```python
from build123d import *

# Parameters (mm, degrees)
BOSS_EXTRUDE1_DEPTH = 25.4
SKETCH2_R           = 1.0287
BOSS_EXTRUDE2_DEPTH = 6.35
SKETCH3_R           = 1.0287
CUT_EXTRUDE1_DEPTH  = 6.35


with BuildPart() as part:
    # Sketch1 → Boss-Extrude1 (new body)
    with BuildSketch(Plane(origin=(0, 0, 0), x_dir=(1, 0, 0), z_dir=(0, 1, 0))):
        with BuildLine():
            Line((-1.135922533, 2.413), (1.135922533, 2.413))
            ThreePointArc((1.135922533, 2.413), (1.3335, 2.309689752), (1.521758033, 2.19023777))
            Line((1.521758033, 2.19023777), (2.657680566, 0.22276223))
            ThreePointArc((2.657680566, 0.22276223), (2.667, 0), (2.657680566, -0.22276223))
            Line((2.657680566, -0.22276223), (1.521758033, -2.19023777))
            ThreePointArc((1.521758033, -2.19023777), (1.3335, -2.309689752), (1.135922533, -2.413))
            Line((1.135922533, -2.413), (-1.135922533, -2.413))
            ThreePointArc((-1.135922533, -2.413), (-1.3335, -2.309689752), (-1.521758033, -2.19023777))
            Line((-1.521758033, -2.19023777), (-2.657680566, -0.22276223))
            ThreePointArc((-2.657680566, -0.22276223), (-2.667, 0), (-2.657680566, 0.22276223))
            Line((-2.657680566, 0.22276223), (-1.521758033, 2.19023777))
            ThreePointArc((-1.521758033, 2.19023777), (-1.3335, 2.309689752), (-1.135922533, 2.413))
        make_face()
    extrude(amount=BOSS_EXTRUDE1_DEPTH)

    # Sketch2 → Boss-Extrude2 (add)
    with BuildSketch(Plane(origin=(0, 25.4, 0), x_dir=(1, 0, 0), z_dir=(0, 1, 0))):
        Circle(SKETCH2_R)
    extrude(amount=BOSS_EXTRUDE2_DEPTH)

    # Sketch3 → Cut-Extrude1 (cut)
    with BuildSketch(Plane.XZ):
        Circle(SKETCH3_R)
    extrude(amount=-CUT_EXTRUDE1_DEPTH, mode=Mode.SUBTRACT)


solid = part.part
```
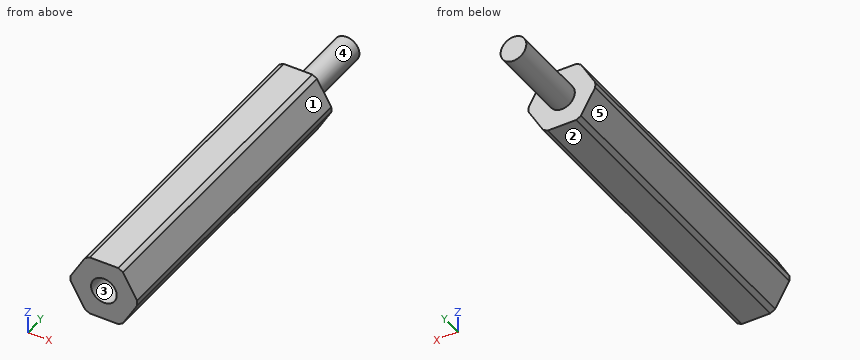
Part model, mm, in its own coordinate system. Face numbers are marked on the shaded views. A direction names the side the tool comes from. Coordinates: 2 decimals unless noted, no trailing zeros. Order: outer loops, then holes, each group sorted by start corner. A loop starts at its lowest first (then second) coordinate and runs counter-clockwise, first axis right, second up. Notation, with made-up numbers: (78.25, 74.25) - (121.25, 74.25) arc R14 ccw to (121.25, 91.25) - close; hole circle Ø9 at (81.25, 4.5). An arc over 180 degrees is marked (long way). Return JSON: item names as keys, results as strings. Group by question number.
Item 1: Pin check, flat tips, straight feed: pin 1 (1.5 mm diameter, centred on y = 9.5, z = 1.5, fed in from +X); pin 2 (1.9 mm diameter, centred on x = 0, z = 0, fed in from -Y). Stop position of each tip, or through.
Item 2: Cut at C-C (z = -1.9). List the corners of the cut face in (x, y), plus the area to 3 significant figures.
Item 3: Drill centre lines: probe 1 along Z at (x, y) = (0, 3.5); probe 2 along Y at (x, z) = (-1.75, 0.15); probe 3 along Y at (x, z) = (-0.1, -0.4). Where is each one in solid material? Low to high. Write a range as from..to.
Item 4: Cut at D-D (y = 29). List the corners of the cut face in (x, z), plus the area to 3 significant figures.
Item 5: Cut at A-A (x = 0). List the corners of the cut face in (y, z).
Item 6: Which spindle directions (+Z, -Z, +X, -X, +Y, -Y) get a long thin tool onto all of the face, cutting with end or side? Do the marked faces 4 and 5. Say none if no direction does.
Item 7: Cut at B-B (y = 15.5). List the corners of the cut face in (x, z), plus the area to 3 significant figures.
Item 8: Pull direction X, two halves, no side cores. Call the marked faces 1, 2 and 3: pulls with the +X half, pulls with the -X half, needs draft (parallel to the pull), parting line crosses it, or undercut.
Check values:
{
 "1": {"pin 1": "stops at x = 2.35", "pin 2": "stops at y = 6.35"},
 "2": {"outline": "(-1.69, 0) - (1.69, 0) - (1.69, 25.4) - (-1.69, 25.4) - close", "area": "85.8 mm2"},
 "3": {"probe 1": "z = -2.41..-1.03, 1.03..2.41", "probe 2": "y = 0..25.4", "probe 3": "y = 6.35..31.75"},
 "4": {"outline": "circle Ø2.06 at (0, 0)", "area": "3.32 mm2"},
 "5": {"outline": "(0, -2.41) - (25.4, -2.41) - (25.4, -1.03) - (31.75, -1.03) - (31.75, 1.03) - (25.4, 1.03) - (25.4, 2.41) - (0, 2.41) - (0, 1.03) - (6.35, 1.03) - (6.35, -1.03) - (0, -1.03) - close"},
 "6": {"face 4": "+Y", "face 5": "-Z, -X, +Y, -Y"},
 "7": {"outline": "(-2.66, -0.22) - (-1.52, -2.19) arc R2.67 ccw to (-1.14, -2.41) - (1.14, -2.41) arc R2.67 ccw to (1.52, -2.19) - (2.66, -0.22) arc R2.67 ccw to (2.66, 0.22) - (1.52, 2.19) arc R2.67 ccw to (1.14, 2.41) - (-1.14, 2.41) arc R2.67 ccw to (-1.52, 2.19) - (-2.66, 0.22) arc R2.67 ccw to start", "area": "20.0 mm2"},
 "8": {"face 1": "pulls with the +X half", "face 2": "needs draft", "face 3": "undercut"}
}
